For this review, take the finished solid that the model builds, in its own axes (mm). A direction names the side the tool comes from. Coordinates: 2 decimals unless noted, no trailing zeros. Order: outer loops, then holes, each group sorted by start corner. A loop starts at its lowest first (then second) coordinate and runs counter-clockwise, first axis right, second up.
from build123d import *

# Parameters (mm, degrees)
SKETCH1_R               = 50.8
BOSS_EXTRUDE1_DEPTH     = 3.175
SKETCH2_R               = 50.8
SKETCH2_R_2             = 44.45
BOSS_EXTRUDE2_DEPTH     = 19.05
SKETCH5_W               = 50.8
SKETCH5_H               = 6.35
BOSS_EXTRUDE3_DEPTH     = 25.4
SKETCH6_W               = 1.5875
SKETCH6_H               = 6.35
CUT_EXTRUDE1_DEPTH      = 6.35
SKETCH7_W               = 19.05
SKETCH7_H               = 25.4
CUT_EXTRUDE2_DEPTH      = 51.8
CUT_EXTRUDE2_DEPTH_BACK = 51.8
SKETCH8_W               = 57.15
SKETCH8_H               = 12.7
CUT_EXTRUDE3_DEPTH      = 51.8
BOSS_EXTRUDE4_DEPTH     = 57.15
SKETCH10_W              = 6.35
SKETCH10_H              = 3.175
BOSS_EXTRUDE5_DEPTH     = 3.175
SKETCH11_W              = 3.175
SKETCH11_H              = 6.35
BOSS_EXTRUDE6_DEPTH     = 12.7
SKETCH12_W              = 63.5
SKETCH12_H              = 6.35
BOSS_EXTRUDE7_DEPTH     = 12.7
SKETCH14_W              = 6.35
SKETCH14_H              = 12.7
BOSS_EXTRUDE8_DEPTH     = 31.75
BOSS_EXTRUDE9_DEPTH     = 9.525


with BuildPart() as part:
    # Sketch1 → Boss-Extrude1 (new body)
    with BuildSketch(Plane(origin=(0, 0, 0), x_dir=(1, 0, 0), z_dir=(0, 1, 0))):
        with Locations(Location((0, 0, 0), (0, 0, 270))):  # turned: the seam where the file's is
            Circle(SKETCH1_R)
    extrude(amount=-BOSS_EXTRUDE1_DEPTH)

    # Sketch2 → Boss-Extrude2 (add)
    with BuildSketch(Plane(origin=(0, 0, 0), x_dir=(1, 0, 0), z_dir=(0, 1, 0))):
        with Locations(Location((0, 0, 0), (0, 0, 270))):  # turned: the seam where the file's is
            Circle(SKETCH2_R)
        with Locations(Location((0, 0, 0), (0, 0, 270))):  # turned: the seam where the file's is
            Circle(SKETCH2_R_2, mode=Mode.SUBTRACT)
    extrude(amount=BOSS_EXTRUDE2_DEPTH)

    # Sketch3 → Revolve3 (revolve)
    with BuildSketch(Plane.XY, mode=Mode.PRIVATE) as revolve3_sk:
        Polygon((44.45, 19.05), (44.45, 25.4), (47.625, 19.05), align=None)
    revolve(revolve3_sk.sketch.rotate(Axis((0, 6.35, 0), (0, -1, 0)), 90), axis=Axis((0, 6.35, 0), (0, -1, 0)))  # turned: the seam where the file's is

    # Sketch5 → Boss-Extrude3 (add)
    with BuildSketch(Plane(origin=(0, 0, 0), x_dir=(1, 0, 0), z_dir=(0, 1, 0))):
        with Locations((0, -19.05)):
            Rectangle(SKETCH5_W, SKETCH5_H)
    extrude(amount=BOSS_EXTRUDE3_DEPTH)

    # Sketch6 → Cut-Extrude1 (cut)
    with BuildSketch(Plane(origin=(0, 25.4, 0), x_dir=(1, 0, 0), z_dir=(0, 1, 0))):
        with Locations((-21.43125, -19.05)):
            Rectangle(SKETCH6_W, SKETCH6_H)
        with Locations((21.43125, -19.05)):
            Rectangle(SKETCH6_W, SKETCH6_H)
    cut_extrude1 = extrude(amount=-CUT_EXTRUDE1_DEPTH, mode=Mode.SUBTRACT)

    # Sketch7 → Cut-Extrude2 (cut, two sides)
    with BuildSketch(Plane(origin=(0, 0, 0), x_dir=(0, 0, -1), z_dir=(1, 0, 0))) as cut_extrude2_sk:
        with Locations((0, 12.7)):
            Rectangle(SKETCH7_W, SKETCH7_H)
    extrude(amount=CUT_EXTRUDE2_DEPTH, mode=Mode.SUBTRACT)
    extrude(cut_extrude2_sk.sketch, amount=-CUT_EXTRUDE2_DEPTH_BACK, mode=Mode.SUBTRACT)

    # Sketch8 → Cut-Extrude3 (cut, through all)
    with BuildSketch(Plane.XY):
        with Locations((0, 6.35)):
            Rectangle(SKETCH8_W, SKETCH8_H)
    extrude(amount=-CUT_EXTRUDE3_DEPTH, mode=Mode.SUBTRACT)

    # Sketch9 → Boss-Extrude4 (add)
    with BuildSketch(Plane(origin=(0, 0, 0), x_dir=(1, 0, 0), z_dir=(0, 1, 0))):
        with BuildLine():
            Line((-28.575, 34.048081811), (-28.575, 30.74349878))
            ThreePointArc((-28.575, 30.74349878), (-36.310709707, 21.05292623), (-40.877472001, 9.525))
            Line((-40.877472001, 9.525), (-43.417472001, 9.525))
            ThreePointArc((-43.417472001, 9.525), (-38.027284831, 23.015823001), (-28.575, 34.048081811))
        make_face()
        with BuildLine():
            Line((28.575, 34.048081811), (28.575, 30.74349878))
            ThreePointArc((28.575, 30.74349878), (36.310709707, 21.05292623), (40.877472001, 9.525))
            Line((40.877472001, 9.525), (43.417472001, 9.525))
            ThreePointArc((43.417472001, 9.525), (38.027284831, 23.015823001), (28.575, 34.048081811))
        make_face()
    extrude(amount=BOSS_EXTRUDE4_DEPTH)

    # Sketch10 → Boss-Extrude5 (add)
    with BuildSketch(Plane(origin=(0, 0, 15.875), x_dir=(-1, 0, 0), z_dir=(0, 0, -1))):
        with Locations((0, 11.1125)):
            Rectangle(SKETCH10_W, SKETCH10_H)
    extrude(amount=BOSS_EXTRUDE5_DEPTH)

    # Sketch11 → Boss-Extrude6 (add)
    with BuildSketch(Plane(origin=(0, 0, 0), x_dir=(1, 0, 0), z_dir=(0, 1, 0))):
        with Locations((-30.1625, 19.05)):
            Rectangle(SKETCH11_W, SKETCH11_H)
        with Locations((30.1625, 19.05)):
            Rectangle(SKETCH11_W, SKETCH11_H)
    extrude(amount=BOSS_EXTRUDE6_DEPTH)

    # Sketch12 → Boss-Extrude7 (add)
    with BuildSketch(Plane(origin=(0, 12.7, 0), x_dir=(1, 0, 0), z_dir=(0, 1, 0))):
        with Locations((0, 19.05)):
            Rectangle(SKETCH12_W, SKETCH12_H)
    extrude(amount=BOSS_EXTRUDE7_DEPTH)

    # Mirror1: Cut-Extrude1 across plane
    add(cut_extrude1.mirror(Plane.XY), mode=Mode.SUBTRACT)

    # Sketch14 → Boss-Extrude8 (add)
    with BuildSketch(Plane.XY.offset(-15.875)):
        with Locations((0, 19.05)):
            Rectangle(SKETCH14_W, SKETCH14_H)
    extrude(amount=BOSS_EXTRUDE8_DEPTH)

    # Sketch15 → Boss-Extrude9 (add)
    with BuildSketch(Plane(origin=(0, 0, 0), x_dir=(1, 0, 0), z_dir=(0, 1, 0))):
        with BuildLine():
            Line((-49.899041824, 9.525), (-43.417472001, 9.525))
            ThreePointArc((-43.417472001, 9.525), (-44.45, 0), (-43.417472001, -9.525))
            Line((-43.417472001, -9.525), (-49.899041824, -9.525))
            ThreePointArc((-49.899041824, -9.525), (-50.8, 0), (-49.899041824, 9.525))
        make_face()
        with BuildLine():
            Line((43.417472001, 9.525), (49.899041824, 9.525))
            ThreePointArc((49.899041824, 9.525), (50.8, 0), (49.899041824, -9.525))
            Line((49.899041824, -9.525), (43.417472001, -9.525))
            ThreePointArc((43.417472001, -9.525), (44.45, 0), (43.417472001, 9.525))
        make_face()
    extrude(amount=BOSS_EXTRUDE9_DEPTH)


solid = part.part
1. To check wall thickness, follow L1, parallel to X at y = 3.5, z = -22 (3 decimals); L2, parallel to X at y = 29, z = -32.5 (3 decimals); L3, parallel to Y at x = 2.5, z = -45.5 (3 decimals). State the ranges of each line that lie inside material, in increasing order.
Answer below:
L1: x = -45.789 to -35.745, -31.75 to -28.575, 28.575 to 31.75, 35.745 to 45.789
L2: x = -30.324 to -28.575, 28.575 to 30.324
L3: y = -3.175 to 0, 12.7 to 23.163
2. Clearance check with flat-ended pins moving along their axes: pin 1 Ø1.9 at (y, z) = (22, 19.5) entering from -X; pin 2 Ø2 at (x, z) = (-14.5, 7.5) entering from +Y; pin 3 Ø6 at (y, z) = (49, -6) entering from +X; pin 4 Ø7.5 at (x, y) = (-17, 12) entering from +Z. State where each tip first meets the part, or that it passes through.
Answer below:
pin 1: stops at x = -42.51
pin 2: stops at y = 0
pin 3: passes through
pin 4: stops at z = 49.04
3. Take a section at C-C, the plane y = 7.5. Give the number of separate pieces and of enclosed holes in the cut face, plus the area to 3 significant figures.
Answer below:
separate pieces: 4
enclosed holes: 0
area: 2,010 mm2
4. The part is to be moulded in two halves that separate along X. For faces 1 (the face through (-8, 18, -22.225)), 2 (the face through (0, 19.05, 48)), 3 (the face through (-38.133, 41.053, -22.841)), say which applies: +X half, -X half, draft (parallel to the pull), parting line (faces both ways), or undercut.
Answer below:
face 1: undercut
face 2: draft
face 3: -X half
5. Take a section at D-D, the plane x = 0. Give the boundary of the cut face in (y, z) (3 decimals), plus the area to 3 significant figures.
Answer below:
outline: (-3.175, -50.8) - (0, -50.8) - (0, 15.875) - (9.525, 15.875) - (9.525, 12.7) - (12.7, 12.7) - (12.7, -22.225) - (25.4, -22.225) - (25.4, 22.225) - (0, 22.225) - (0, 44.45) - (25.4, 44.45) - (19.05, 47.625) - (19.05, 50.8) - (-3.175, 50.8) - close; (12.7, -50.8) - (19.05, -50.8) - (19.05, -47.625) - (25.4, -44.45) - (12.7, -44.45) - close
area: 1,160 mm2
6. Take a section at B-B, the plane z = 0. Give the boundary of the cut face in (x, y) (3 decimals), plus the area to 3 significant figures.
Answer below:
outline: (-50.8, -3.175) - (50.8, -3.175) - (50.8, 9.525) - (44.45, 9.525) - (44.45, 0) - (-44.45, 0) - (-44.45, 9.525) - (-50.8, 9.525) - close; (-3.175, 12.7) - (3.175, 12.7) - (3.175, 25.4) - (-3.175, 25.4) - close
area: 524 mm2
7. Machinability: for faces 4 (the face through (0, 12.7, -14)), 5 (the face through (-28.575, 22, -33)), 6 (the face through (20.638, 22, -19)), which of the approach directions +Z, -Z, +X, -X, +Y, -Y give a long, thin tool a straight path to every point of the face, cutting with its end or side? Answer none if there is none.
Answer below:
face 4: -Z
face 5: none
face 6: +Y
